Job drawing, mm, ordinate dimensions from the low corner. One solid piece. A direction names the side the tool comes from. Coordinates: 2 decimals unless noted, no trailing zeros. Order: outer loops, then holes, each group sorted by start corner. A loop starts at its lowest first (then second) coordinate and runs counter-clockwise, first axis right, second up. Notation, with made-up numbers: M 55,76 L 68,76 A13 ccw 68,98 Z; hole C -32,-13.75 d5. An arc over 180 degrees is marked long. Write item = value, one per line. Start each with the question number.
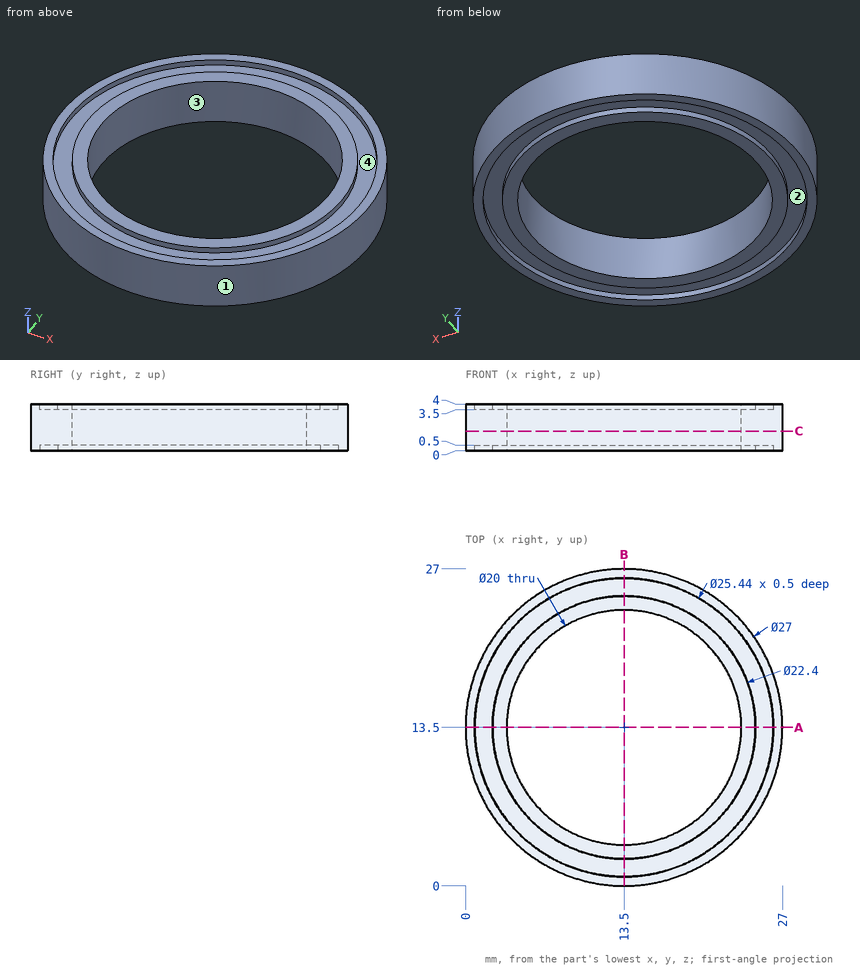
Item 1: Wall check: line 1 along Y through (x, z) = (13.5, 0.45); line 2 along X through (y, z) = (21.5, 3.7); line 3 along Y through (x, z) = (20, 3.7). Give the ranges that are in metal, low to high. Write a range as [from, to].
Item 2: Cut at A-A, the plane y = 13.5. Write the cut outline in (x, z).
Item 3: 3-axis set-ups, long thin cutter, end or side, ignore diameter. For the marked faces 3 and 4: which of +Z, -Z, +X, -X, +Y, -Y reach the whole face in a straight line?
Item 4: Flat gauge pin, fed straight in: pin 1 (1.5 mm diameter, centred on x = 6.5, y = 4, fed in from -Z). Where does the tip first touch, or does it go through?
Item 5: Cut at C-C, the plane z = 1.7. Write the cut outline in (x, y), and give its area (3 significant figures).
Item 6: Pull direction X, two halves, no side cores. Call the marked faces 1 and 2: pulls with the +X half, pulls with the -X half, needs draft (parallel to the pull), parting line crosses it, or undercut.
Filled sheet:
q1.line_1 = [0, 0.78], [2.3, 3.5], [23.5, 24.7], [26.22, 27]
q1.line_2 = [2.63, 3.61], [5.66, 7.5], [19.5, 21.34], [23.39, 24.37]
q1.line_3 = [1.67, 2.57], [4.38, 5.9], [21.1, 22.62], [24.43, 25.33]
q2.outline = M 0,0 L 0.78,0 L 0.78,0.5 L 2.3,0.5 L 2.3,0 L 3.5,0 L 3.5,4 L 2.3,4 L 2.3,3.5 L 0.78,3.5 L 0.78,4 L 0,4 Z; M 23.5,0 L 24.7,0 L 24.7,0.5 L 26.22,0.5 L 26.22,0 L 27,0 L 27,4 L 26.22,4 L 26.22,3.5 L 24.7,3.5 L 24.7,4 L 23.5,4 Z
q3.face_3 = +Z, -Z
q3.face_4 = +Z
q4.pin_1 = 0
q5.outline = C 13.5,13.5 d27; hole C 13.5,13.5 d20
q5.area = 258 mm2
q6.face_1 = parting line crosses it
q6.face_2 = undercut
